```python
from build123d import *

# Parameters (mm, degrees)
ESQUISSE1_W        = 105
ESQUISSE1_H        = 105
ESQUISSE1_R        = 1.25
ESQUISSE1_R_2      = 1.65
BOSS_EXTRU_1_DEPTH = 5
CONG_1_R           = 5


with BuildPart() as part:
    # Esquisse1 → Boss.-Extru.1 (new body)
    with BuildSketch(Plane.XY):
        with Locations((52.5, 52.5)):
            Rectangle(ESQUISSE1_W, ESQUISSE1_H)
        with Locations((5.5, 5.5)):
            Circle(ESQUISSE1_R, mode=Mode.SUBTRACT)
        with Locations(Location((99.5, 5.5, 0), (0, 0, 180))):
            Circle(ESQUISSE1_R, mode=Mode.SUBTRACT)
        with Locations((99.5, 99.5)):
            Circle(ESQUISSE1_R, mode=Mode.SUBTRACT)
        with Locations(Location((5.5, 99.5, 0), (0, 0, 180))):
            Circle(ESQUISSE1_R, mode=Mode.SUBTRACT)
        with Locations((22.5, 67.5)):
            Circle(ESQUISSE1_R_2, mode=Mode.SUBTRACT)
        with Locations(Location((22.5, 37.5, 0), (0, 0, 180))):
            Circle(ESQUISSE1_R_2, mode=Mode.SUBTRACT)
        with Locations((82.5, 37.5)):
            Circle(ESQUISSE1_R_2, mode=Mode.SUBTRACT)
        with Locations(Location((82.5, 67.5, 0), (0, 0, 180))):
            Circle(ESQUISSE1_R_2, mode=Mode.SUBTRACT)
    extrude(amount=BOSS_EXTRU_1_DEPTH)

    # Congé1
    cong_1_edges = [part.edges().sort_by_distance(p)[0] for p in [
        (0, 105, 2.5),
        (105, 105, 2.5),
        (105, 0, 2.5),
        (0, 0, 2.5),
    ]]
    fillet(cong_1_edges, radius=CONG_1_R)


solid = part.part
```
Check sheet for the modelled part. Datum: model origin and axes. Units: mm. Give positions to 0.01 mm unless a question says otherwise; leave off trailing zeros. Write each loop counter-clockwise with the first axis right and the second up, starting at its lowest first coordinate (ties: lowest second). Pieces come first, ordered by that corner, then holes. Notation, with made-up numbers: (66.5, -3) - (97.5, -3) arc R33 ccw to (97.5, 31) - close; hole circle Ø4 at (17, 31.25). An arc over 180 degrees is marked (long way). Answer as a JSON object with one key per item and string values. Group by question number.
1) Thickness scan on probe 1 along X at (y, z) = (67.5, 1.75); probe 2 along Y at (x, z) = (99.5, 3.5); probe 3 along Y at (x, z) = (22.5, 1.3). Record the ranges inside material, lowest first. Write a range as from..to.
2) Sectioned sample at A-A (x = 82.5). Record the cut outline in (y, z), then the cut area to 3 significant figures.
3) Sectioned sample at B-B (y = 67.5). Record the cut outline in (x, z).
4) Depth check by flat-ended pin: P1, Ø4, axis at x = 5.5, y = 99.5, coming from the -Z side. Enter the tip coordinate at first touch or a pass-through.
5) Release check for a two-part mould opening along Y. For faces 1 (the face through (52, 105, 2)), 2 (the face through (52, 53, 0)), 3 (the face through (5.23, 4.28, 2.46)) record: pulls with the +Y half, pulls with the -Y half, needs draft (parallel to the pull), parting line crosses it, or undercut.
Geometry results:
{
 "1": {"probe 1": "x = 0..20.85, 24.15..80.85, 84.15..105", "probe 2": "y = 0..4.25, 6.75..98.25, 100.75..105", "probe 3": "y = 0..35.85, 39.15..65.85, 69.15..105"},
 "2": {"outline": "(0, 0) - (35.85, 0) - (35.85, 5) - (0, 5) - close; (39.15, 0) - (65.85, 0) - (65.85, 5) - (39.15, 5) - close; (69.15, 0) - (105, 0) - (105, 5) - (69.15, 5) - close", "area": "492 mm^2"},
 "3": {"outline": "(0, 0) - (20.85, 0) - (20.85, 5) - (0, 5) - close; (24.15, 0) - (80.85, 0) - (80.85, 5) - (24.15, 5) - close; (84.15, 0) - (105, 0) - (105, 5) - (84.15, 5) - close"},
 "4": {"P1": "stops at z = 0"},
 "5": {"face 1": "pulls with the +Y half", "face 2": "needs draft", "face 3": "undercut"}
}
